Input: part model. Units: mm. Frame: model coordinates. Give positions to 0.01 mm unless a question says otherwise; leave off trailing zeros. Loops run counter-clockwise (first coordinate to the right, second up) from the corner with the lowest first, then second, coordinate; pieces in that order, holes last. Notation, with made-up numbers: M 86.25,-4.75 L 94.25,-4.75 A16 cw 94.25,4.25 Z; hole C -34,-34 d9. An arc over 180 degrees is marked long. Answer as a JSON object with one key per item and string values. Group by question number.
1) Section query B-B on z = 14.5. Return loops of the section in (x, y).
2) Section query A-A on z = 34.5. Return loops of the section in (x, y).
3) First-contact query: P1, Ø1, axis at y = 1.5, z = -20, coming from the +X side; P2, Ø5, axis at x = -42.57, z = 14.5, coming from the +Y side; P3, Ø0.6, axis at x = 21.5, y = 0.5, coming from the +Z side; P4, Ø0.6, axis at y = 0.5, z = -5.5, coming from the +X side. Flat tips, straight axial feed; report the tip coordinate or a pass-through.
4) Ray query, L1, parallel to Z at x = -40, y = 0.9; L2, parallel to Z at x = -8, y = 1.6; L3, parallel to X at y = 1.3, z = -5.5. Return the intervals inside material, ascending.
5) Section query D-D on z = -34.5. Return loops of the section in (x, y).
6) Section query C-C on x = -32. Return loops of the section in (y, z).
from build123d import *

# Parameters (mm, degrees)
SKETCH1_R           = 2.1
SKETCH1_R_2         = 9
SKETCH1_W           = 11
SKETCH1_H           = 2.8
BOSS_EXTRUDE2_DEPTH = 2
FILLET2_R           = 2
FILLET3_R           = 2
FILLET4_R           = 2
FILLET5_R           = 2


with BuildPart() as part:
    # Sketch1 → Boss-Extrude2 (new body)
    with BuildSketch(Plane(origin=(0, 0, 0), x_dir=(1, 0, 0), z_dir=(0, 1, 0))):
        with BuildLine():
            Line((-37.900233161, -45.013744243), (-37.900233161, -56.220541455))
            ThreePointArc((-37.900233161, -56.220541455), (-67.973978104, 0.144116575), (-37.900233161, 56.508774605))
            Line((-37.900233161, 56.508774605), (-37.900233161, 45.013744243))
            Line((-37.900233161, 45.013744243), (16.055748962, 44.986255757))
            Line((16.055748962, 44.986255757), (16.055748962, 42.486255757))
            Line((16.055748962, 42.486255757), (27.055748962, 42.486255757))
            Line((27.055748962, 42.486255757), (27.055748962, 44.986255757))
            Line((27.055748962, 44.986255757), (40.223874261, 44.986255757))
            Line((40.223874261, 44.986255757), (40.223874261, 54.986255757))
            ThreePointArc((40.223874261, 54.986255757), (68.16767133, -0.013744243), (40.223874261, -55.013744243))
            Line((40.223874261, -55.013744243), (40.223874261, -45.013744243))
            Line((40.223874261, -45.013744243), (27.055748962, -45.013744243))
            Line((27.055748962, -45.013744243), (27.055748962, -42.465581387))
            Line((27.055748962, -42.465581387), (16.055748962, -42.465581387))
            Line((16.055748962, -42.465581387), (16.055748962, -45.013744243))
            Line((16.055748962, -45.013744243), (-37.900233161, -45.013744243))
        make_face()
        with Locations(Location((40.004613264, -34.516033797, 0), (0, 0, 270))):
            Circle(SKETCH1_R, mode=Mode.SUBTRACT)
        with Locations(Location((40.000233161, 34.5, 0), (0, 0, 90))):
            Circle(SKETCH1_R, mode=Mode.SUBTRACT)
        with Locations(Location((37.900233161, -14.5, 0), (0, 0, 270))):
            Circle(SKETCH1_R, mode=Mode.SUBTRACT)
        with Locations(Location((37.900233161, 14.5, 0), (0, 0, 90))):
            Circle(SKETCH1_R, mode=Mode.SUBTRACT)
        with Locations(Location((60.900233161, 14.5, 0), (0, 0, 270))):
            Circle(SKETCH1_R, mode=Mode.SUBTRACT)
        with Locations(Location((60.900233161, -14.5, 0), (0, 0, 90))):
            Circle(SKETCH1_R, mode=Mode.SUBTRACT)
        with Locations(Location((-40.000233161, -34.5, 0), (0, 0, 90))):
            Circle(SKETCH1_R, mode=Mode.SUBTRACT)
        with Locations(Location((-35.900233161, -14.5, 0), (0, 0, 90))):
            Circle(SKETCH1_R, mode=Mode.SUBTRACT)
        with Locations(Location((-58.900233161, -14.5, 0), (0, 0, 270))):
            Circle(SKETCH1_R, mode=Mode.SUBTRACT)
        with Locations(Location((-58.900233161, 14.5, 0), (0, 0, 90))):
            Circle(SKETCH1_R, mode=Mode.SUBTRACT)
        with Locations(Location((-35.900233161, 14.5, 0), (0, 0, 270))):
            Circle(SKETCH1_R, mode=Mode.SUBTRACT)
        with Locations(Location((-40.000233161, 34.5, 0), (0, 0, 270))):
            Circle(SKETCH1_R, mode=Mode.SUBTRACT)
        with Locations(Location((26.366427779, -0.013744243, 0), (0, 0, 270))):
            Circle(SKETCH1_R_2, mode=Mode.SUBTRACT)
        with Locations(Location((-37.900233161, 0, 0), (0, 0, 270))):
            Circle(SKETCH1_R_2, mode=Mode.SUBTRACT)
        with Locations(Location((28.973777757, -14.234221967, 0), (0, 0, 270))):
            Circle(SKETCH1_R, mode=Mode.SUBTRACT)
        with Locations(Location((28.973777757, 14.5, 0), (0, 0, 90))):
            Circle(SKETCH1_R, mode=Mode.SUBTRACT)
        with Locations(Location((28.973777757, 34.770177046, 0), (0, 0, 270))):
            Circle(SKETCH1_R, mode=Mode.SUBTRACT)
        with Locations(Location((-42.568753496, -14.5, 0), (0, 0, 270))):
            Circle(SKETCH1_R, mode=Mode.SUBTRACT)
        with Locations(Location((-42.568753496, 14.5, 0), (0, 0, 90))):
            Circle(SKETCH1_R, mode=Mode.SUBTRACT)
        Polygon((-17.02036954, 21.11975573), (-17.019395908, 18.319755899), (-7.019396513, 18.323233156), (-7.020370144, 21.123232986), align=None, mode=Mode.SUBTRACT)
        with Locations((21.555748962, -22.565581387)):
            Rectangle(SKETCH1_W, SKETCH1_H, mode=Mode.SUBTRACT)
        with Locations((21.555748962, 22.5380929)):
            Rectangle(SKETCH1_W, SKETCH1_H, mode=Mode.SUBTRACT)
        Polygon((-17.022091972, -4.030680267), (-17.022315971, -6.830680258), (-7.022316003, -6.831480257), (-7.022092004, -4.031480266), align=None, mode=Mode.SUBTRACT)
        Polygon((-17.02036954, 4.02323402), (-7.020370144, 4.019756764), (-7.019396513, 6.819756595), (-17.019395908, 6.823233851), align=None, mode=Mode.SUBTRACT)
        Polygon((-17.029404589, -21.127200413), (-7.029407596, -21.134954923), (-7.027236333, -18.334955765), (-17.027233326, -18.327201255), align=None, mode=Mode.SUBTRACT)
    extrude(amount=BOSS_EXTRUDE2_DEPTH)

    # Fillet2
    fillet2_edges = [part.edges().sort_by_distance(p)[0] for p in [
        (-37.900233161, 1, -56.508774605),
    ]]
    fillet(fillet2_edges, radius=FILLET2_R)

    # Fillet3
    fillet3_edges = [part.edges().sort_by_distance(p)[0] for p in [
        (40.223874261, 1, -54.986255757),
    ]]
    fillet(fillet3_edges, radius=FILLET3_R)

    # Fillet4
    fillet4_edges = [part.edges().sort_by_distance(p)[0] for p in [
        (40.223874261, 1, 55.013744243),
    ]]
    fillet(fillet4_edges, radius=FILLET4_R)

    # Fillet5
    fillet5_edges = [part.edges().sort_by_distance(p)[0] for p in [
        (-37.900233161, 1, 56.220541455),
    ]]
    fillet(fillet5_edges, radius=FILLET5_R)


solid = part.part
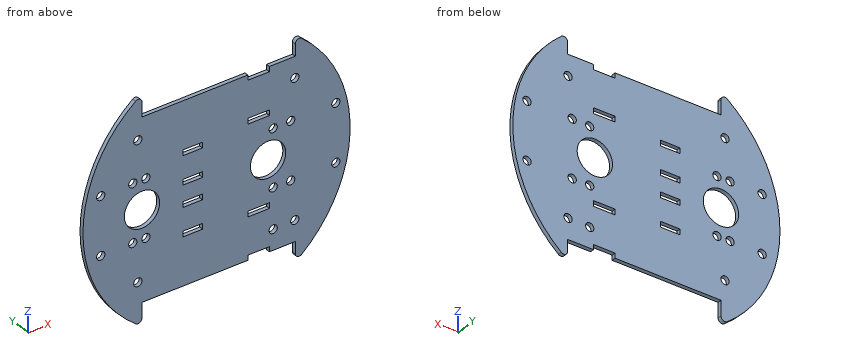
Output:
{
 "1": {"outline": "M -66.37,0 L -61,0 L -61,2 L -66.37,2 Z; M -56.8,0 L -44.67,0 L -44.67,2 L -56.8,2 Z; M -40.47,0 L -38,0 L -38,2 L -40.47,2 Z; M -33.8,0 L 26.89,0 L 26.89,2 L -33.8,2 Z; M 31.06,0 L 35.8,0 L 35.8,2 L 31.06,2 Z; M 40,0 L 58.8,0 L 58.8,2 L 40,2 Z; M 63,0 L 66.61,0 L 66.61,2 L 63,2 Z"},
 "2": {"outline": "M -58.46,0 L -42.1,0 L -42.1,2 L -58.46,2 Z; M -37.9,0 L 37.9,0 L 37.9,2 L -37.9,2 Z; M 42.1,0 L 58.79,0 L 58.79,2 L 42.1,2 Z"},
 "3": {"P1": "stops at x = 65.31", "P2": "stops at y = 2", "P3": "stops at z = 42.47", "P4": "stops at x = 67.97"},
 "4": {"L1": "z = -54.62 to -36.6, -32.4 to -8.75, 8.75 to 32.4, 36.6 to 54.34", "L2": "z = -45 to -21.12, -18.32 to -6.82, -4.02 to 4.03, 6.83 to 18.33, 21.13 to 45.01", "L3": "x = -67.76 to -45.02, -30.78 to -17.02, -7.02 to 19.25, 33.48 to 67.94"},
 "5": {"outline": "M -58.63,0 L -42.1,0 L -42.1,2 L -58.63,2 Z; M -37.9,0 L 26.89,0 L 26.89,2 L -37.9,2 Z; M 31.06,0 L 37.9,0 L 37.9,2 L 31.06,2 Z; M 42.1,0 L 58.77,0 L 58.77,2 L 42.1,2 Z"},
 "6": {"outline": "M 0,-45.01 L 2,-45.01 L 2,-6.8 L 0,-6.8 Z; M 0,6.8 L 2,6.8 L 2,45.01 L 0,45.01 Z"}
}
